from build123d import *

# Parameters (mm, degrees)
EXTRUDE_1_DEPTH          = 40
SKETCH_2_R               = 11
CUT_EXTRUDE_1_DEPTH      = 48.602520942
SKETCH_3_R               = 2.4
CUT_EXTRUDE_2_DEPTH      = 8
PATTERN_CIRCULAR_2_COUNT = 8
SKETCH_4_W               = 10
SKETCH_4_H               = 3.367948213
EXTRUDE_2_DEPTH          = 40
SKETCH_5_W               = 3
SKETCH_5_H               = 2
CUT_EXTRUDE_3_DEPTH      = 49.884853937


with BuildPart() as part:
    # 草图1 → 凸台-拉伸1 (new body)
    with BuildSketch(Plane(origin=(0, 0, 0), x_dir=(1, 0, 0), z_dir=(0, 1, 0))):
        with BuildLine():
            Line((-15, 14.696938457), (-15, -14.696938457))
            ThreePointArc((-15, -14.696938457), (0, -21), (15, -14.696938457))
            Line((15, -14.696938457), (15, 14.696938457))
            ThreePointArc((15, 14.696938457), (0, 21), (-15, 14.696938457))
        make_face()
    extrude(amount=EXTRUDE_1_DEPTH)

    # 草图2 → 切除-拉伸1 (cut, through all)
    with BuildSketch(Plane(origin=(0, 40, 0), x_dir=(1, 0, 0), z_dir=(0, 1, 0))):
        with Locations(Location((0, 0, 0), (0, 0, 270))):
            Circle(SKETCH_2_R)
    extrude(amount=-CUT_EXTRUDE_1_DEPTH, mode=Mode.SUBTRACT)

    # 草图3 → 切除-拉伸2 (cut)
    with BuildSketch(Plane(origin=(0, 40, 0), x_dir=(1, 0, 0), z_dir=(0, 1, 0))):
        with Locations(Location((-11.313708499, 11.313708499, 0), (0, 0, 270))):
            Circle(SKETCH_3_R)
    cut_extrude_2 = extrude(amount=-CUT_EXTRUDE_2_DEPTH, mode=Mode.SUBTRACT)

    # 阵列(圆周)2: 切除-拉伸2 ×8 about axis, 2 skipped
    pattern_circular_2_axis = Axis((0, 40, 0), (0, 1, 0))
    add([cut_extrude_2.rotate(pattern_circular_2_axis, i * 360 / PATTERN_CIRCULAR_2_COUNT) for i in range(1, PATTERN_CIRCULAR_2_COUNT) if i not in (1, 5)], mode=Mode.SUBTRACT)

    # 草图4 → 凸台-拉伸2 (add)
    with BuildSketch(Plane(origin=(0, 0, 0), x_dir=(1, 0, 0), z_dir=(0, 1, 0))):
        with Locations((0, -22.080052161)):
            Rectangle(SKETCH_4_W, SKETCH_4_H)
    extrude(amount=EXTRUDE_2_DEPTH)

    # 草图5 → 切除-拉伸3 (cut, through all)
    with BuildSketch(Plane(origin=(0, 0, 0), x_dir=(1, 0, 0), z_dir=(0, 1, 0))):
        with Locations((0, -22.764026267)):
            Rectangle(SKETCH_5_W, SKETCH_5_H)
    extrude(amount=CUT_EXTRUDE_3_DEPTH, mode=Mode.SUBTRACT)


solid = part.part
For this review, take the finished solid that the model builds, in its own axes (mm). A direction names the side the tool comes from. Round coordinates to 2 decimals unless told otherwise and drop trailing zeros. Write each loop counter-clockwise with the first axis right and the second up, starting at its lowest first coordinate (ties: lowest second). Pieces come first, ordered by that corner, then holes. Notation, with made-up numbers: (83.25, 75) - (119.25, 75) arc R26 ccw to (119.25, 104) - close; hole circle Ø11 at (73, -7.5). An arc over 180 degrees is marked (long way). Write item = value, one per line. Start each with the question number.
1. Draft analysis for pull direction X (two halves, no side actions). For faces 4 (the face through (15, 20, 0)), 5 (the face through (0, 32, -16)), 6 (the face through (-15, 20, 0)), 7 (the face through (-1.5, 20, 23)), state which applies: released by +X, released by -X, zero draft, split by the parting line, or undercut.
2. Consider section B-B on x = 0. State the section outline as (y, z) points.
3. Consider section A-A on z = 0. State the section outline as (x, y) points, plus the area to 3 significant figures.
4. For pin 1 Ø5 at (x, y) = (-12, 32) entering from +Z; pin 2 Ø2 at (y, z) = (20, 23) entering from +X; pin 3 Ø1.4 at (x, z) = (10.5, 12) entering from +Y, all flat-tipped, find the tip position at first contact; note any pin that passes through.
5. Wall thickness on L1, parallel to Y at x = -13, z = 11.5; L2, parallel to Z at x = -10, y = 14; L3, parallel to X at y = 3, z = -9.5: over which ranges is each line inside the solid? List them lowest first.
6. For faces 1 (the face through (5, 20, 22)), 2 (the face through (-5, 20, 22)), 3 (the face through (0, 20, 21.764)), list the 3-axis set-ups (+Z, -Z, +X, -X, +Y, -Y) from which the entire face can be reached by the end or side of a thin tool; tool diameter is ignored.
7. Consider section D-D on z = 21. State the section outline as (x, y) points, plus the area to 3 significant figures.
8. Consider section C-C on y = 21. State the section outline as (x, z) points.
Evaluation:
q1.face_4 = released by +X
q1.face_5 = undercut
q1.face_6 = released by -X
q1.face_7 = undercut
q2.outline = (0, -21) - (40, -21) - (40, -18.4) - (32, -18.4) - (32, -13.6) - (40, -13.6) - (40, -11) - (0, -11) - close; (0, 11) - (40, 11) - (40, 13.6) - (32, 13.6) - (32, 18.4) - (40, 18.4) - (40, 21.76) - (0, 21.76) - close
q3.outline = (-15, 0) - (-11, 0) - (-11, 40) - (-15, 40) - close; (11, 0) - (15, 0) - (15, 40) - (11, 40) - close
q3.area = 320 mm2
q4.pin_1 = 18.73
q4.pin_2 = 5
q4.pin_3 = 32
q5.L1 = 0 to 32
q5.L2 = -18.47 to -4.58, 4.58 to 18.47
q5.L3 = -15 to -5.55, 5.55 to 15
q6.face_1 = +Z, +X, +Y, -Y
q6.face_2 = +Z, -X, +Y, -Y
q6.face_3 = +Z, +Y, -Y
q7.outline = (-5, 0) - (5, 0) - (5, 40) - (-5, 40) - close
q7.area = 400 mm2
q8.outline = (-15, -14.7) arc R21 ccw to (15, -14.7) - (15, 14.7) arc R21 ccw to (5, 20.4) - (5, 23.76) - (1.5, 23.76) - (1.5, 21.76) - (-1.5, 21.76) - (-1.5, 23.76) - (-5, 23.76) - (-5, 20.4) arc R21 ccw to (-15, 14.7) - close; hole circle Ø22 at (0, 0)
